from build123d import *

# Parameters (mm, degrees)
SKETCH1_W           = 40.26
SKETCH1_H           = 20
BOSS_EXTRUDE1_DEPTH = 36.86
SKETCH2_W           = 20
SKETCH2_H           = 2.6
BOSS_EXTRUDE2_DEPTH = 7.17
SKETCH3_W           = 20
SKETCH3_H           = 2.6
BOSS_EXTRUDE3_DEPTH = 7.17
SKETCH4_R           = 10
BOSS_EXTRUDE4_DEPTH = 2.48
SKETCH5_R           = 6.55
BOSS_EXTRUDE5_DEPTH = 1.56
SKETCH6_R           = 2.9
BOSS_EXTRUDE6_DEPTH = 4.2
SKETCH7_W           = 40.26
SKETCH7_H           = 20
CUT_EXTRUDE1_DEPTH  = 15


with BuildPart() as part:
    # Sketch1 → Boss-Extrude1 (new body)
    with BuildSketch(Plane(origin=(0, 0, 0), x_dir=(1, 0, 0), z_dir=(0, 1, 0))):
        Rectangle(SKETCH1_W, SKETCH1_H)
    extrude(amount=BOSS_EXTRUDE1_DEPTH)

    # Sketch2 → Boss-Extrude2 (add)
    with BuildSketch(Plane(origin=(20.13, 0, 0), x_dir=(0, 0, -1), z_dir=(1, 0, 0))):
        with Locations((0, 29.3)):
            Rectangle(SKETCH2_W, SKETCH2_H)
    extrude(amount=BOSS_EXTRUDE2_DEPTH)

    # Sketch3 → Boss-Extrude3 (add)
    with BuildSketch(Plane.ZY.offset(20.13)):
        with Locations((0, 29.3)):
            Rectangle(SKETCH3_W, SKETCH3_H)
    extrude(amount=BOSS_EXTRUDE3_DEPTH)

    # Sketch4 → Boss-Extrude4 (add)
    with BuildSketch(Plane(origin=(0, 36.86, 0), x_dir=(1, 0, 0), z_dir=(0, 1, 0))):
        with Locations((-10.13, 0)):
            Circle(SKETCH4_R)
        with BuildLine():
            Line((13.87, 10), (-10.13, 10))
            ThreePointArc((-10.13, 10), (-3.058932188, 7.071067812), (-0.13, 0))
            ThreePointArc((-0.13, 0), (-3.058932188, -7.071067812), (-10.13, -10))
            Line((-10.13, -10), (13.87, -10))
            Line((13.87, -10), (13.87, 10))
        make_face()
    extrude(amount=BOSS_EXTRUDE4_DEPTH)

    # Sketch5 → Boss-Extrude5 (add)
    with BuildSketch(Plane(origin=(0, 39.34, 0), x_dir=(1, 0, 0), z_dir=(0, 1, 0))):
        with Locations((-10.13, 0)):
            Circle(SKETCH5_R)
    extrude(amount=BOSS_EXTRUDE5_DEPTH)

    # Sketch6 → Boss-Extrude6 (add)
    with BuildSketch(Plane(origin=(0, 40.9, 0), x_dir=(1, 0, 0), z_dir=(0, 1, 0))):
        with Locations((-10.13, 0)):
            Circle(SKETCH6_R)
    extrude(amount=BOSS_EXTRUDE6_DEPTH)

    # Sketch7 → Cut-Extrude1 (cut)
    with BuildSketch(Plane.XZ):
        Rectangle(SKETCH7_W, SKETCH7_H)
    extrude(amount=-CUT_EXTRUDE1_DEPTH, mode=Mode.SUBTRACT)


solid = part.part
The listing builds one solid part. Answer for the finished solid, in the listing's coordinates (mm). A direction names the side the tool comes from. Coordinates: 2 decimals unless noted, no trailing zeros. Write each loop counter-clockwise with the first axis right and the second up, starting at its lowest first coordinate (ties: lowest second). Pieces come first, ordered by that corner, then holes. Notation, with made-up numbers: (-4.75, -11.75) - (37.25, -11.75) arc R13 cw to (37.25, -1.75) - close; hole circle Ø2 at (-24, 42). An arc over 180 degrees is marked (long way). Answer as CSV lines item,"result".
1. Straight lines are drawn through the part: line 1 (Y direction, x = -7, z = -1); line 2 (X direction, y = 20.5, z = 4.75); line 3 (Y direction, x = 11, z = 4.5). For each, find the intervals that lie inside material, in ascending order. Write a range as [from, to].
Computed values:
line 1,"y = [15, 40.9]"
line 2,"x = [-20.13, 20.13]"
line 3,"y = [15, 39.34]"
2. A tool of negligible diameter and unlimited length cuts with its end or side. For faces 1 (the flat face through (20.13, 34, 0)), 2 (the flat face through (-7, 40.9, 1)), 3 (the flat face through (-20.13, 34, 0)), from which of +Z, -Z, +X, -X, +Y, -Y can it reach the whole face along a straight path? Write none if from no direction.
Computed values:
face 1,"+Z, -Z, +X, +Y"
face 2,"+Y"
face 3,"+Z, -Z, -X, +Y"
3. Find section D-D (z = -8.5). Give the vertices of the cut face in (x, y), plus the area to 3 significant figures.
Computed values:
outline,"(-27.3, 28) - (-20.13, 28) - (-20.13, 15) - (20.13, 15) - (20.13, 28) - (27.3, 28) - (27.3, 30.6) - (20.13, 30.6) - (20.13, 36.86) - (13.87, 36.86) - (13.87, 39.34) - (-15.4, 39.34) - (-15.4, 36.86) - (-20.13, 36.86) - (-20.13, 30.6) - (-27.3, 30.6) - close"
area,"990 mm²"
4. Given P1, Ø1, axis at y = 20.5, z = 2.5, coming from the -X side; P2, Ø8, axis at x = -16.5, z = 7, coming from the +Y side; P3, Ø3.5, axis at x = -25, z = 4, coming from the +Y side; P4, Ø10.5, axis at x = -12.5, z = 2, coming from the +Y side, each flat-ended and moving along its own axis, determine where each tip first touches the part or whether it passes through.
Computed values:
P1,"stops at x = -20.13"
P2,"stops at y = 40.9"
P3,"stops at y = 30.6"
P4,"stops at y = 45.1"
5. Find section B-B (z = -4). Give the vertices of the cut face in (x, y).
Computed values:
outline,"(-27.3, 28) - (-20.13, 28) - (-20.13, 15) - (20.13, 15) - (20.13, 28) - (27.3, 28) - (27.3, 30.6) - (20.13, 30.6) - (20.13, 36.86) - (13.87, 36.86) - (13.87, 39.34) - (-4.94, 39.34) - (-4.94, 40.9) - (-15.32, 40.9) - (-15.32, 39.34) - (-19.3, 39.34) - (-19.3, 36.86) - (-20.13, 36.86) - (-20.13, 30.6) - (-27.3, 30.6) - close"
6. Find section A-A (x = -21). Give the vertices of the cut face in (y, z).
Computed values:
outline,"(28, -10) - (30.6, -10) - (30.6, 10) - (28, 10) - close"
7. Find section C-C (y = 34). Give the vertices of the cut face in (x, z), plus the area to 3 significant figures.
Computed values:
outline,"(-20.13, -10) - (20.13, -10) - (20.13, 10) - (-20.13, 10) - close"
area,"805 mm²"
